Here's how the part is built. I have some questions about the finished solid (model axes, mm). A direction names the side the tool comes from. Round coordinates to 2 decimals unless told otherwise and drop trailing zeros. Write each loop counter-clockwise with the first axis right and the second up, starting at its lowest first coordinate (ties: lowest second). Pieces come first, ordered by that corner, then holes. Notation, with made-up numbers: M 52.5,71 L 93.5,71 A15 ccw 93.5,87 Z; hole C 83,43 d8. An arc over 180 degrees is marked long. Use a Markdown table: item, result. Add a question column.
```python
from build123d import *

# Parameters (mm, degrees)
SKETCH_1_W          = 20
SKETCH_1_H          = 12
SKETCH_1_R          = 0.625
SKETCH_1_R_2        = 1.525
SKETCH_1_R_3        = 2.525
EXTRUDE_1_DEPTH     = 2
SKETCH_3_R          = 0.7
CUT_EXTRUDE_1_DEPTH = 24.409399821
SKETCH_3_3_R        = 1
CUT_EXTRUDE_2_DEPTH = 1.5


with BuildPart() as part:
    # Sketch 1 → Extrude 1 (new body)
    with BuildSketch(Plane(origin=(0, 0, 0), x_dir=(1, 0, 0), z_dir=(0, 1, 0))):
        with Locations((10, -6)):
            Rectangle(SKETCH_1_W, SKETCH_1_H)
        with Locations(Location((9.732863826, -4.1, 0), (0, 0, 270))):
            Circle(SKETCH_1_R, mode=Mode.SUBTRACT)
        with Locations(Location((10.350101922, -9.120648628, 0), (0, 0, 270))):
            Circle(SKETCH_1_R_2, mode=Mode.SUBTRACT)
        with Locations(Location((6.331393556, -7.9, 0), (0, 0, 270))):
            Circle(SKETCH_1_R, mode=Mode.SUBTRACT)
        with Locations(Location((15, -6, 0), (0, 0, 270))):
            Circle(SKETCH_1_R_3, mode=Mode.SUBTRACT)
    extrude(amount=EXTRUDE_1_DEPTH)

    # Sketch 3 → Cut-Extrude 1 (cut, through all)
    with BuildSketch(Plane(origin=(0, 2, 0), x_dir=(1, 0, 0), z_dir=(0, 1, 0))):
        with Locations(Location((1.101301337, -10.801482832, 0), (0, 0, 270))):
            Circle(SKETCH_3_R)
        with Locations(Location((1.310630289, -4.626278754, 0), (0, 0, 270))):
            Circle(SKETCH_3_R)
        with Locations(Location((18.067159924, -1.34892989, 0), (0, 0, 270))):
            Circle(SKETCH_3_R)
        with Locations(Location((18.067159924, -10.801482832, 0), (0, 0, 270))):
            Circle(SKETCH_3_R)
    extrude(amount=-CUT_EXTRUDE_1_DEPTH, mode=Mode.SUBTRACT)

    # Sketch 3_3 → Cut-Extrude 2 (cut)
    with BuildSketch(Plane(origin=(0, 2, 0), x_dir=(1, 0, 0), z_dir=(0, 1, 0))):
        with Locations(Location((1.310630289, -4.626278754, 0), (0, 0, 270))):
            Circle(SKETCH_3_3_R)
        with Locations(Location((1.101301337, -10.801482832, 0), (0, 0, 270))):
            Circle(SKETCH_3_3_R)
        with Locations(Location((18.067159924, -1.34892989, 0), (0, 0, 270))):
            Circle(SKETCH_3_3_R)
        with Locations(Location((18.067159924, -10.801482832, 0), (0, 0, 270))):
            Circle(SKETCH_3_3_R)
    extrude(amount=-CUT_EXTRUDE_2_DEPTH, mode=Mode.SUBTRACT)


solid = part.part
```
Item 1: I need wall thicknesses on probe 1 along X at (y, z) = (1.3, 4.25); probe 2 along Z at (x, y) = (9.5, 1.2); probe 3 along X at (y, z) = (1.65, 5). Which ranges of each line are inside material? Lowest first, please. Write a range as from..to.
Item 2: Imagine slicing it at C-C on y = 0.9. Count the separate pieces of the cut face and the enclosed holes in it, plus the area to 3 significant figures.
Item 3: Imagine slicing it at D-D on z = 7.9. List the corners of the cut face in (x, y) for me.
Item 4: Imagine slicing it at B-B on x = 15. List the corners of the cut face in (y, z) for me (3 decimals).
Item 5: For pin 1 Ø1.8 at (x, z) = (18.07, 1.35) entering from +Y, with a flat end and sliding along its axis, tell me the tip position at first contact or that it passes through.
Item 6: On a 3-axis mill with a long thin cutter (end or side, diameter ignored), from which of +Z, -Z, +X, -X, +Y, -Y can I reach the whole of each face in a straight line? I mean faces 5 (the face through (19.06, 1.26, 10.67)), 6 (the face through (10, 0, 6)). Say none if no direction works.
Item 7: Imagine slicing it at A-A on z = 6. List the corners of the cut face in (x, y) for me (3 decimals), plus the area to 3 significant figures.
Item 8: If we mould it in two halves opening along X, with no side actions, what happens to faces 1 (the face through (20, 1, 6)), 2 (the face through (10, 1, 0)), 3 (the face through (1.341, 0.254, 3.927)), 4 (the face through (0, 1, 6))? For each: +X half, -X half, draft (parallel to the pull), parting line (faces both ways), or undercut.
The answers:
| question | item | result |
|---|---|---|
| 1 | probe 1 | 0..0.38, 2.24..9.13, 10.34..13.18, 16.82..20 |
| 1 | probe 2 | 0..3.52, 4.68..7.85, 10.39..12 |
| 1 | probe 3 | 0..0.38, 2.24..12.68, 17.32..20 |
| 2 | separate pieces | 1 |
| 2 | enclosed holes | 8 |
| 2 | area | 198 mm² |
| 3 | outline | M 0,0 L 5.71,0 L 5.71,2 L 0,2 Z; M 6.96,0 L 9.44,0 L 9.44,2 L 6.96,2 Z; M 11.26,0 L 13.34,0 L 13.34,2 L 11.26,2 Z; M 16.66,0 L 20,0 L 20,2 L 16.66,2 Z |
| 4 | outline | M 0,0 L 2,0 L 2,3.475 L 0,3.475 Z; M 0,8.525 L 2,8.525 L 2,12 L 0,12 Z |
| 5 | pin 1 | y = 0.5 |
| 6 | face 5 | +Y |
| 6 | face 6 | +Z, -Z, +X, -X, -Y |
| 7 | outline | M 0,0 L 12.475,0 L 12.475,2 L 0,2 Z; M 17.525,0 L 20,0 L 20,2 L 17.525,2 Z |
| 7 | area | 29.9 mm² |
| 8 | face 1 | +X half |
| 8 | face 2 | draft |
| 8 | face 3 | undercut |
| 8 | face 4 | -X half |
